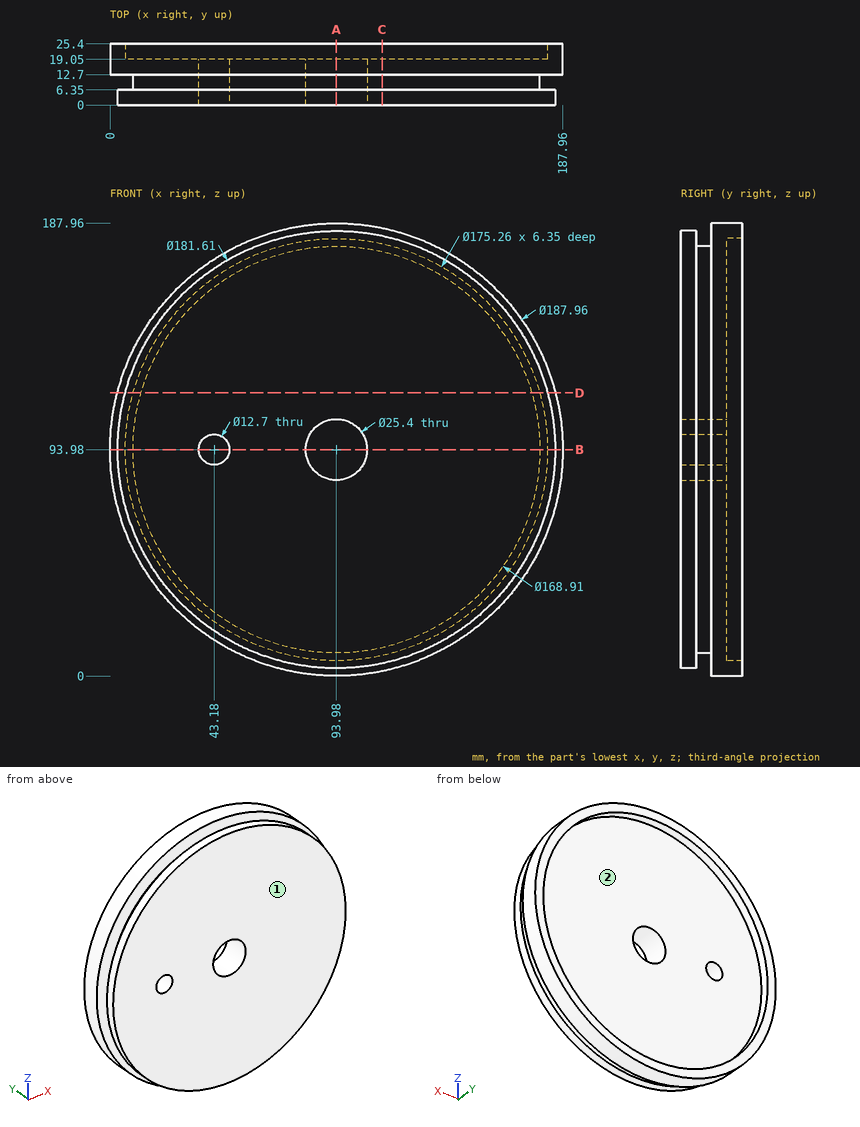
Print and shaded views of the part. All mm, measured from the part's lowest x, y and z. Give positions to 0.01 mm unless a question says otherwise; leave off trailing zeros. Order: outer loops, then holes, each group sorted by start corner. A loop starts at its lowest first (then second) coordinate and runs counter-clockwise, first axis right, second up. Notation, with made-up numbers: (4, -6.5) - (29, -6.5) arc R17 cw to (29, 14.5) - close; hole circle Ø1 at (74.5, -22). An arc over 180 degrees is marked (long way). Use a Markdown table: item, result.
1) Saw through at D-D on z = 117.5. List the corners of the cut face in (x, y).
Checked values:
| item | result |
|---|---|
| outline | (2.99, 12.7) - (12.87, 12.7) - (12.87, 6.35) - (6.27, 6.35) - (6.27, 0) - (181.69, 0) - (181.69, 6.35) - (175.09, 6.35) - (175.09, 12.7) - (184.97, 12.7) - (184.97, 25.4) - (178.39, 25.4) - (178.39, 19.05) - (9.57, 19.05) - (9.57, 25.4) - (2.99, 25.4) - close |
2) Saw through at B-B on z = 93.98. List the corners of the cut face in (x, y) (3 decimals).
Checked values:
| item | result |
|---|---|
| outline | (0, 12.7) - (9.525, 12.7) - (9.525, 6.35) - (3.175, 6.35) - (3.175, 0) - (36.83, 0) - (36.83, 19.05) - (6.35, 19.05) - (6.35, 25.4) - (0, 25.4) - close; (49.53, 0) - (81.28, 0) - (81.28, 19.05) - (49.53, 19.05) - close; (106.68, 0) - (184.785, 0) - (184.785, 6.35) - (178.435, 6.35) - (178.435, 12.7) - (187.96, 12.7) - (187.96, 25.4) - (181.61, 25.4) - (181.61, 19.05) - (106.68, 19.05) - close |
3) Flat gauge pins, fed straight in: P1, Ø5, axis at x = 75.5, z = 167, coming from the +Y side; P2, Ø12, axis at y = 15.5, z = 124, coming from the -X side; P3, Ø11.5, axis at x = 43.18, z = 93.98, coming from the +Y side; P4, Ø4, axis at x = 133, y = 3, coming from the +Z side. Where does each tip first touch, or does it go through?
Checked values:
| item | result |
|---|---|
| P1 | y = 19.05 |
| P2 | x = 3.12 |
| P3 | through |
| P4 | z = 176.9 |
4) Probe L1, parallel to X at y = 9.5, z = 93.98 (3 decimals); L2, parallel to Z at x = 93.98, y = 22.5; L3, parallel to Y at x = 84, z = 84. List the from-to ranges inside material, lowest first. Write a range as from..to.
Checked values:
| item | result |
|---|---|
| L1 | 9.525..36.83, 49.53..81.28, 106.68..178.435 |
| L2 | 0..6.35, 181.61..187.96 |
| L3 | 0..19.05 |
5) Two-plate mould, pull along Z, no slides. Class the marked faces 1 and 2: +Z half, -Z half, draft (parallel to the pull), parting line (faces both ways), or undercut.
Checked values:
| item | result |
|---|---|
| face 1 | draft |
| face 2 | undercut |
6) Saw through at A-A on x = 93.98. List the corners of the cut face in (y, z) (3 decimals), plus the area to 3 significant figures.
Checked values:
| item | result |
|---|---|
| outline | (0, 3.175) - (6.35, 3.175) - (6.35, 9.525) - (12.7, 9.525) - (12.7, 0) - (25.4, 0) - (25.4, 6.35) - (19.05, 6.35) - (19.05, 81.28) - (0, 81.28) - close; (0, 106.68) - (19.05, 106.68) - (19.05, 181.61) - (25.4, 181.61) - (25.4, 187.96) - (12.7, 187.96) - (12.7, 178.435) - (6.35, 178.435) - (6.35, 184.785) - (0, 184.785) - close |
| area | 3,020 mm² |
7) Saw through at C-C on x = 113. List the corners of the cut face in (y, z), plus the area to 3 significant figures.
Checked values:
| item | result |
|---|---|
| outline | (0, 5.19) - (6.35, 5.19) - (6.35, 11.69) - (12.7, 11.69) - (12.7, 1.94) - (25.4, 1.94) - (25.4, 8.44) - (19.05, 8.44) - (19.05, 179.52) - (25.4, 179.52) - (25.4, 186.02) - (12.7, 186.02) - (12.7, 176.27) - (6.35, 176.27) - (6.35, 182.77) - (0, 182.77) - close |
| area | 3,420 mm² |
